Autodesk Fusion 360 part; units mm, degrees
sketch "holder" plane through (0, 0, 0) normal (0, 0, 1) x (-1, 0, 0)
  line L0 (6, -16.5) -> (18.75, -16.5)
  line L1 (18.75, 0) -> (6, 0)
  line L2 (23.8137, -14.7632) -> (21.6655, -12)
  line L3 (21.6655, -4.5) -> (23.8137, -1.7368)
  line L4 (21.6655, -12) -> (18.75, -8.25) construction
  line L5 (18.75, -8.25) -> (21.6655, -4.5) construction
  line L6 (18.75, -8.25) -> (21.6655, -8.25) construction
  line L7 (21.6655, -8.25) -> (21.6655, -12) construction
  line L8 (21.6655, -8.25) -> (21.6655, -4.5) construction
  line L9 (18.75, -8.25) -> (13, -8.25) construction
  arc A0 (18.75, -16.5) -> (23.8137, -14.7632) centre (18.75, -8.25) ccw
  arc A1 (23.8137, -1.7368) -> (18.75, 0) centre (18.75, -8.25) ccw
  arc A2 (22.2793, -3.7105) -> (22.2793, -12.7895) centre (18.75, -8.25) ccw
  arc A3 (21.6655, -4.5) -> (21.6655, -12) centre (18.75, -8.25) ccw
  line L10 (6, -16.5) -> (0, -16.5)
  line L11 (0, -16.5) -> (0, 0)
  line L12 (0, 0) -> (6, 0)
  line L13 (6, -16.5) -> (6, 0)
  dimension "d49" = 11.5
  dimension "d50" = 9.5
  dimension "d51" = 7.5
  dimension "d63" = 6
  dimension "d64" = 13
  dimension "d65" = 16.5
extrude "Extrude4" add sketch "holder" against normal blind 8 contours L0 L1 L2 L3 A0 A1 A2 L13
extrude "Extrude5" add sketch "holder" against normal blind 3 from surface at -8 contours L0 L1 L2 L3 A0 A1 A2 L13 | L2 L3 A2 A3
chamfer "Chamfer4" distance 1 angle 45 1 edges at (-13, 8.25, -8)
sketch "screws" plane through (-6, 0, 0) normal (1, 0, 0) x (0, 1, 0)
  line L0 (16.5, 0) -> (0, 0)
  line L1 (0, 0) -> (0, -11)
  line L2 (0, -11) -> (16.5, -11)
  line L3 (16.5, -11) -> (16.5, 0)
  circle A0 centre (8.25, -16) radius 2.25
  circle A1 centre (8.25, -16) radius 5
  circle A2 centre (8.25, -28.25) radius 2.25
  circle A3 centre (8.25, -28.25) radius 5
  line L4 (8.25, -16) -> (8.25, -28.25) construction
  line L5 (8.25, -16) -> (8.25, -11) construction
  line L6 (0, 0) -> (0, -28.25)
  arc A4 (0, -28.25) -> (16.5, -28.25) centre (8.25, -28.25) ccw
  line L7 (16.5, -28.25) -> (16.5, 0)
  line L8 (0, 0) -> (16.5, 0)
  point P0 (8.25, -11)
  dimension "d77" = 4.5
  dimension "d78" = 10
  dimension "d79" = 12.25
extrude "Extrude7" add sketch "screws" along normal blind 6 contours L0 L1 L2 L3 L6 L7 L8 | A1 | L2 L6 A4 L7 | A3
chamfer "Chamfer5" distance 2.75 angle 45 2 edges at (-6, 6.1523, -15.1864) (-6, 6.1523, -27.4364)
chamfer "Chamfer6" distance 1 angle 45 10 edges at (-6, 16.5, -19.625) (-6, 0, -19.625) (-6, 8.25, -36.5) (-12.375, 16.5, -11) (-21.4267, 16.0537, -11) (-22.7396, 13.3816, -11) (-14, 8.25, -11) (-22.7396, 3.1184, -11) (-12.375, 0, -11) (-21.4267, 0.4463, -11)
fillet "Fillet5" radius 0.5 6 edges at (-23.8137, 14.7632, -5) (-22.2793, 12.7895, -3.5) (-21.9724, 12.3947, -7.5) (-22.2793, 3.7105, -3.5) (-23.8137, 1.7368, -5) (-21.9724, 4.1053, -7.5)
equation "d49 = largeD"
equation "d50 = smallD"
equation "d51 = opening"
equation "d63 = mountT"
equation "d64 = largeProjection"
equation "d65 = width"
equation "screwOuterD = 10 mm"
equation "screwInnerD = 4.5 mm"
equation "smallD = ( largeD + opening ) / 2"
equation "largeD = 11.5 mm"
equation "opening = 7.5 mm"
equation "largeProjection = 13 mm"
equation "width = largeD + 5 mm"
equation "sheathH = 8 mm"
equation "d76 = ( largeD - smallD ) / 2"
equation "d77 = screwInnerD"
equation "d78 = screwOuterD"
equation "d79 = screwOuterD + screwInnerD / 2"
equation "mountT = 6 mm"
equation "d81 = mountT"
equation "d83 = ( screwOuterD - screwInnerD ) / 2"
equation "lipH = 3 mm"
Geometry check sheet. Reference: the model listing, model coordinates, mm. A direction names the side the tool comes from. Round coordinates to 2 decimals unless told otherwise and drop trailing zeros. Loops run counter-clockwise (first coordinate to the right, second up) from the corner with the lowest first, then second, coordinate; pieces in that order, holes last. Notation, with made-up numbers: M 28.5,-33 L 62.5,-33 A19 ccw 62.5,-10 Z; hole C -38,-40 d10. An arc over 180 degrees is marked long. Return JSON: item names as keys, results as strings. Group by question number.
(1) Go/stop test with flat-tipped pins: pin 1 (8 mm diameter, centred on y = 4, z = -17, fed in from -X); pin 2 (4.5 mm diameter, centred on x = -14.5, y = 8, fed in from -Z). Record where each tip stops, or that it passes through.
(2) Section check B-B, the plane z = -9.5. Enter the section's corners in (x, y).
(3) Section check A-A, the plane z = -16. Enter the section's corners in (x, y), and give its area (3 significant figures).
(4) Section check C-C, the plane y = 7.75. Give the number of separate pieces and of enclosed holes in the cut face, and give its area (3 significant figures).
(5) Mould release check, pull along Z, two halves, no side actions. Record for faces 1 (the face through (-9, 8, 0)), 2 (the face through (-21.2, 0.9, -10.5)), 3 (the face through (-1.648, 7.762, -26.054)): pulls with the +Z half, pulls with the -Z half, needs draft (parallel to the pull), parting line crosses it, or undercut.
(6) Set-up check for faces 4 (the face through (-11.8, 16, -10.5)), 5 (the face through (-22.4, 2.9, -10.4)), 6 (the face through (-22.8, 13.46, -6.04)), 7 (the face through (-12, 0.5, -10.5)), 8 (the face through (-13.8, 8.1, -7.8)): record each of +Z, -Z, +X, -X, +Y, -Y from which the full face is reachable in a straight line by a thin tool's end or side.
(7) Scan lines: line 1 along Z through (x, y) = (-1.35, 8.25); line 2 along Y through (x, z) = (-18.75, -3); line 3 along Z through (x, y) = (-11.25, 8.75). Record each from-to range of solid material in increasing order. Write a range as [from, to].
Data:
{
 "1": {"pin 1": "x = -6", "pin 2": "z = -11"},
 "2": {"outline": "M -23.5,2.14 A0.5 ccw -23.38,1.42 A8.25 ccw -18.75,0 L 0,0 L 0,16.5 L -18.75,16.5 A8.25 ccw -23.38,15.08 A0.5 ccw -23.5,14.36 L -21.67,12 A4.75 cw long -21.67,4.5 Z"},
 "3": {"outline": "M -6,1 L -5,0 L 0,0 L 0,6 L -3.25,6 L -6,3.25 Z; M -6,13.25 L -3.25,10.5 L 0,10.5 L 0,16.5 L -5,16.5 L -6,15.5 Z", "area": "63.4 mm²"},
 "4": {"separate pieces": "3", "enclosed holes": "0", "area": "231 mm²"},
 "5": {"face 1": "pulls with the +Z half", "face 2": "pulls with the -Z half", "face 3": "undercut"},
 "6": {"face 4": "-Z, -X, +Y", "face 5": "-Z, -X", "face 6": "+Z, -Z, -X", "face 7": "-Z, -X, -Y", "face 8": "+Z"},
 "7": {"line 1": "[-36.5, -30.5], [-26, -18.25], [-13.75, 0]", "line 2": "[0, 2.5], [14, 16.5]", "line 3": "[-11, 0]"}
}
